For this review, take the finished solid that the model builds, in its own axes (mm). A direction names the side the tool comes from. Round coordinates to 2 decimals unless told otherwise and drop trailing zeros. Loops run counter-clockwise (first coordinate to the right, second up) from the corner with the lowest first, then second, coordinate; pieces in that order, holes last. Notation, with made-up numbers: (0.5, 13.5) -> (37.5, 13.5) arc R27 ccw to (37.5, 45.5) -> close; hole circle Ø4 at (-30, -39.5). An arc over 180 degrees is marked (long way). One line per question, with ' | ' between items. Start each with the question number.
1. Consider section B-B (x = -4.5). Write out the cut boundary in (y, z), and give its area (3 significant figures).
2. For faces 1 (the face through (-2.5, 10, 286)), 2 (the face through (0, 9, 286)), list the 3-axis set-ups (+Z, -Z, +X, -X, +Y, -Y) from which the entire face can be reached by the end or side of a thin tool; tool diameter is ignored.
3. Consider section A-A (z = 150). Write out the cut boundary in (x, y).
4. Wall thickness on line 1 along Y through (x, z) = (-1, 370); line 2 along Z through (x, y) = (-0.5, 11.5); line 3 along Z through (x, y) = (-1.25, 8.25): over which ranges is each line inside the solid? List them lowest first.
5. For pin 1 Ø5 at (y, z) = (10, 210) entering from -X; pin 2 Ø3 at (y, z) = (15, 201.5) entering from +X; pin 3 Ø4 at (x, z) = (-5.5, 317.5) entering from +Y, all flat-tipped, find the tip position at first contact; note any pin that passes through.
```python
from build123d import *

# Parameters (mm, degrees)
EXTRUDE_1_DEPTH    = 580
HOLE_WIZARD_M5_1_D = 4.2


with BuildPart() as part:
    # 草图1 → 凸台-拉伸1 (new body)
    with BuildSketch(Plane.XY):
        Polygon((0, 0), (0, 18), (-2.5, 18), (-2.5, 2), (-7.5, 2), (-7.5, 0), align=None)
    extrude(amount=EXTRUDE_1_DEPTH)

    # M5 螺纹孔1 (through all)
    with Locations(Plane.ZY.offset(2.5)):
        with Locations((130, 10), (210, 10), (370, 10), (450, 10)):
            Hole(HOLE_WIZARD_M5_1_D / 2)


solid = part.part
```
Answer block:
1) outline: (0, 0) -> (2, 0) -> (2, 580) -> (0, 580) -> close | area: 1,160 mm2
2) face 1: +Z, -Z, -X, +Y | face 2: +Z, -Z, +X, +Y, -Y
3) outline: (-7.5, 0) -> (0, 0) -> (0, 18) -> (-2.5, 18) -> (-2.5, 2) -> (-7.5, 2) -> close
4) line 1: y = 0 to 7.9, 12.1 to 18 | line 2: z = 0 to 128.53, 131.47 to 208.53, 211.47 to 368.53, 371.47 to 448.53, 451.47 to 580 | line 3: z = 0 to 128.84, 131.16 to 208.84, 211.16 to 368.84, 371.16 to 448.84, 451.16 to 580
5) pin 1: stops at x = -2.5 | pin 2: stops at x = 0 | pin 3: stops at y = 2
